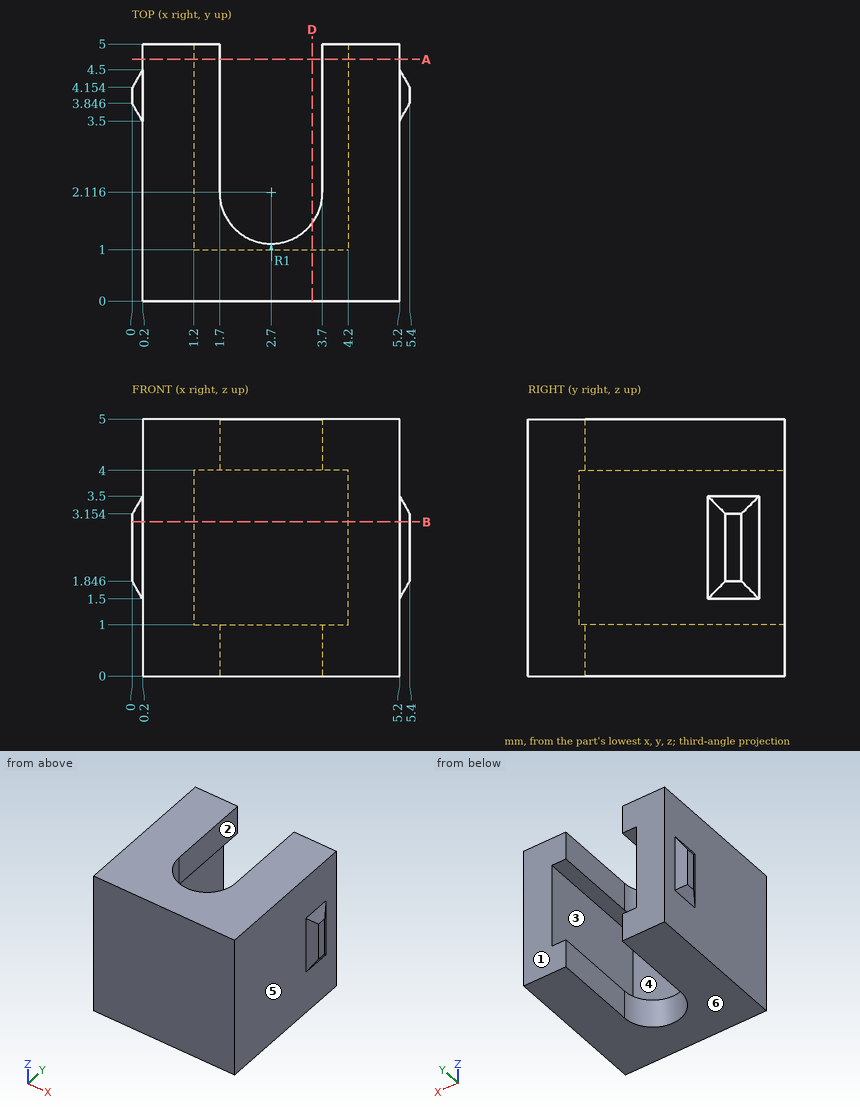
Drawing for the job (mm, zero at the part's lowest x, y, z). A direction names the side the tool comes from. Round coordinates to 2 decimals unless told otherwise and drop trailing zeros. Write each loop counter-clockwise with the first axis right and the second up, starting at its lowest first coordinate (ties: lowest second). Pieces come first, ordered by that corner, then holes. Notation, with made-up numbers: (77.25, 48) - (102.25, 48) arc R20 cw to (102.25, 85) - close; hole circle Ø1 at (39, -17.75). An arc over 180 degrees is marked (long way). Write item = value, one per line. Start each with the question number.
Q1. Probe L1, parallel to X at y = 4.05, z = 2.7; L2, parallel to X at y = 4.1, z = 0.55; L3, parallel to Z at x = 1.25, y = 1.9. List the from-to ranges inside material, lowest first. Write a range as from..to.
Q2. Which spindle directions (+Z, -Z, +X, -X, +Y, -Y) get a long thin tool onto all of the face, cutting with end or side? Do the marked faces 1, 2 and 3. Say none if no direction does.
Q3. Band-saw the part on D-D (x = 3.5). Give the cut face in (y, z) (1 decimal).
Q4. Band-saw the part on B-B (z = 3). Give the cut face in (x, y).
Q5. Band-saw the part on A-A (y = 4.7). Give the cut face in (x, z).
Q6. Mould opens along Z. For the marked faces 4, 5 and 6 say: pulls with the +Z half, pulls with the -Z half, needs draft (parallel to the pull), parting line crosses it, or undercut.
Q7. Drop flat-ended pins along their axis: pin 1 (1.5 mm diameter, centred on x = 2.5, z = 2.5, fed in from +Y); pin 2 (0.8 mm diameter, centred on y = 4, z = 4.5, fed in from +X); pin 3 (1.1 mm diameter, centred on y = 4, z = 4.5, fed in from -X). Give the stop position or say it passes through.
Answers below:
q1.L1 = 0..1.2, 4.2..5.4
q1.L2 = 0.2..1.7, 3.7..5.2
q1.L3 = 0..1, 4..5
q2.face_1 = +Z, -Z, +X, -X, +Y
q2.face_2 = +Z, -Z, +Y
q2.face_3 = +Y
q3.outline = (0, 0) - (1.5, 0) - (1.5, 1) - (1, 1) - (1, 4) - (1.5, 4) - (1.5, 5) - (0, 5) - close
q4.outline = (0, 3.85) - (0.2, 3.5) - (0.2, 0) - (5.2, 0) - (5.2, 3.5) - (5.4, 3.85) - (5.4, 4.15) - (5.2, 4.5) - (5.2, 5) - (4.2, 5) - (4.2, 1) - (1.2, 1) - (1.2, 5) - (0.2, 5) - (0.2, 4.5) - (0, 4.15) - close
q5.outline = (0.2, 0) - (1.7, 0) - (1.7, 1) - (1.2, 1) - (1.2, 4) - (1.7, 4) - (1.7, 5) - (0.2, 5) - close; (3.7, 0) - (5.2, 0) - (5.2, 5) - (3.7, 5) - (3.7, 4) - (4.2, 4) - (4.2, 1) - (3.7, 1) - close
q6.face_4 = undercut
q6.face_5 = needs draft
q6.face_6 = pulls with the -Z half
q7.pin_1 = 1
q7.pin_2 = 5.2
q7.pin_3 = 0.2
